Geometry check sheet. Reference: the model listing, model coordinates, mm. Face numbers are marked on the shaded views. Round coordinates to 2 decimals unless told otherwise and drop trailing zeros. Write each loop counter-clockwise with the first axis right and the second up, starting at its lowest first coordinate (ties: lowest second). Pieces come first, ordered by that corner, then holes. Notation, with made-up numbers: (4.5, -33.5) -> (43.5, -33.5) arc R30 cw to (43.5, -9.5) -> close; hole circle Ø2 at (25.5, 39.25). An arc over 180 degrees is marked (long way). One line per question, with ' | ' between items.
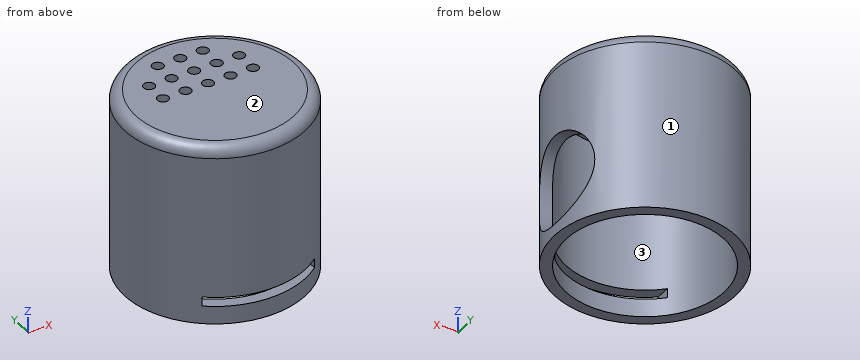
Autodesk Fusion 360 part; units mm, degrees
sketch "スケッチ1" plane through (0, 0, 0) normal (0, 0, 1) x (1, 0, 0)
  circle A0 centre (0, 0) radius 40
extrude "押し出し1" add sketch "スケッチ1" along normal blind 80
shell "シェル1" thickness 5 removed faces 1 at (9.4847, -14.2223, 0)
fillet "フィレット1" radius 5 1 edges at (-37.2931, -14.4646, 80)
ref_plane "作業平面1" through (45, 0, 0) normal (1, 0, 0) x (0, 1, 0)
sketch "スケッチ2" plane through (45, 0, 0) normal (1, 0, 0) x (0, 1, 0)
  circle A0 centre (0, 25) radius 20
extrude "押し出し2" cut sketch "スケッチ2" against normal blind 25
sketch "スケッチ3" plane through (0, 0, 80) normal (0, 0, 1) x (-1, 0, 0)
  circle A0 centre (0, 0) radius 35
  circle A1 centre (10, -25) radius 2.5
  circle A2 centre (0, -25) radius 2.5
  circle A3 centre (-10, -25) radius 2.5
  circle A4 centre (10, -15) radius 2.5
  circle A5 centre (0, -15) radius 2.5
  circle A6 centre (-10, -15) radius 2.5
  circle A7 centre (-20, -15) radius 2.5
  circle A8 centre (20, -15) radius 2.5
  circle A9 centre (0, -5) radius 2.5
  circle A10 centre (-10, -5) radius 2.5
  circle A11 centre (-20, -5) radius 2.5
  circle A12 centre (10, -5) radius 2.5
  circle A13 centre (20, -5) radius 2.5
  dimension "d9" = 5
  dimension "d10" = 5
  dimension "d11" = 5
  dimension "d12" = 5
  dimension "d13" = 5
  dimension "d14" = 5
  dimension "d15" = 5
  dimension "d16" = 5
  dimension "d17" = 5
  dimension "d18" = 5
  dimension "d19" = 5
  dimension "d20" = 5
  dimension "d21" = 5
extrude "押し出し3" cut sketch "スケッチ3" against normal blind 8 contours A1 | A2 | A3 | A4 | A5 | A6 | A7 | A8 | A9 | A10 | A11 | A12 | A13
ref_plane "作業平面2" through (0, -45, 0) normal (0, 1, 0) x (0, 0, 1)
sketch "スケッチ4" plane through (0, -45, 0) normal (0, 1, 0) x (1, 0, 0)
  line L0 (-25, -12.0407) -> (25, -12.0407)
  line L1 (25, -12.0407) -> (25, -7.9593)
  line L2 (25, -7.9593) -> (-25, -7.9593)
  line L3 (-25, -7.9593) -> (-25, -12.0407)
  line L4 (-25, -12.0407) -> (25, -7.9593) construction
  line L5 (25, -12.0407) -> (-25, -7.9593) construction
  point P0 (0, -10)
  dimension "d25" = 50
extrude "押し出し4" cut sketch "スケッチ4" along normal blind 30
(1) Sectioned sample at C-C on x = -10. Count the separate pieces of the cut face and the enclosed holes in it, then the cut area to 3 significant figures.
Resolved:
separate pieces: 5 | enclosed holes: 0 | area: 1,060 mm2
(2) Sectioned sample at A-A on y = 0. Record the cut outline in (x, z).
Resolved:
outline: (-40, 0) -> (-35, 0) -> (-35, 75) -> (35, 75) -> (35, 45) -> (40, 45) -> (40, 75) arc R5 ccw to (35, 80) -> (-35, 80) arc R5 ccw to (-40, 75) -> close; (35, 0) -> (40, 0) -> (40, 5) -> (35, 5) -> close
(3) Draft check along Y on the marked faces 1, 2 and 3. Enter one of: +Y half, -Y half, draft (parallel to the pull), parting line (faces both ways), or undercut.
Resolved:
face 1: parting line | face 2: draft | face 3: undercut
(4) Sectioned sample at B-B on z = 71. Record the cut outline in (x, y), then the cut area to 3 significant figures.
Resolved:
outline: circle Ø80 at (0, 0); hole circle Ø70 at (0, 0) | area: 1,180 mm2
(5) Go/stop test with flat-tipped pins: pin 1 (1.2 mm diameter, centred on y = -28.5, z = 10.5, fed in from -X); pin 2 (6 mm diameter, centred on x = 0, y = 5, fed in from -Z); pin 3 (6 mm diameter, centred on x = -17.5, z = 28, fed in from -Y); pin 4 (4 mm diameter, centred on x = -10, y = 25, fed in from -Z). Record where each tip stops, or that it passes through.
Resolved:
pin 1: stops at x = -28.66 | pin 2: stops at z = 75 | pin 3: stops at y = -37.28 | pin 4: passes through
(6) Material ranges on line 1 (Y direction, x = -10, z = 78); line 2 (Z direction, x = -12.5, y = -33); line 3 (X direction, y = 25, z = 76), recorded low to high.
Resolved:
line 1: y = -37.7 to 2.5, 7.5 to 12.5, 17.5 to 22.5, 27.5 to 37.7 | line 2: z = 0 to 7.96, 12.04 to 79.99 | line 3: x = -31.1 to -12.5, -7.5 to -2.5, 2.5 to 7.5, 12.5 to 31.1
